from build123d import *

# Parameters (mm, degrees)
SKETCH_1_R               = 70
EXTRUDE_1_DEPTH          = 10
SKETCH_3_R               = 105
SKETCH_3_R_2             = 70
EXTRUDE_3_DEPTH          = 30
SKETCH_6_R               = 34
EXTRUDE_4_DEPTH          = 10
SKETCH_7_R               = 22
CUT_EXTRUDE_1_DEPTH      = 30
CUT_EXTRUDE_2_DEPTH      = 20
PATTERN_CIRCULAR_1_COUNT = 6
SKETCH_10_R              = 3
CUT_EXTRUDE_4_DEPTH      = 30
PATTERN_CIRCULAR_2_COUNT = 4
SKETCH_15_R              = 34
CUT_EXTRUDE_6_DEPTH      = 5


with BuildPart() as part:
    # 草图1 → 凸台-拉伸1 (new, symmetric)
    with BuildSketch(Plane(origin=(0, 0, 0), x_dir=(1, 0, 0), z_dir=(0, 1, 0))):
        with Locations(Location((0, 0, 0), (0, 0, 270))):
            Circle(SKETCH_1_R)
    extrude(amount=EXTRUDE_1_DEPTH, both=True)

    # 草图3 → 凸台-拉伸3 (add, symmetric)
    with BuildSketch(Plane(origin=(0, 0, 0), x_dir=(1, 0, 0), z_dir=(0, 1, 0))):
        with Locations(Location((0, 0, 0), (0, 0, 270))):
            Circle(SKETCH_3_R)
        with Locations(Location((0, 0, 0), (0, 0, 270))):
            Circle(SKETCH_3_R_2, mode=Mode.SUBTRACT)
    extrude(amount=EXTRUDE_3_DEPTH, both=True)

    # 草图6 → 凸台-拉伸4 (add)
    with BuildSketch(Plane.XZ.offset(10)):
        with Locations(Location((0, 0, 0), (0, 0, 90))):
            Circle(SKETCH_6_R)
    extrude(amount=EXTRUDE_4_DEPTH)

    # 草图7 → 切除-拉伸1 (cut)
    with BuildSketch(Plane.XZ.offset(20)):
        with Locations(Location((0, 0, 0), (0, 0, 270))):
            Circle(SKETCH_7_R)
    extrude(amount=-CUT_EXTRUDE_1_DEPTH, mode=Mode.SUBTRACT)

    # 草图8 → 切除-拉伸2 (cut)
    with BuildSketch(Plane.XZ.offset(10)):
        with BuildLine():
            Line((-6.945927107, 39.39231012), (-11.287131548, 64.012503946))
            ThreePointArc((-11.287131548, 64.012503946), (0, 65), (11.287131548, 64.012503946))
            Line((11.287131548, 64.012503946), (6.945927107, 39.39231012))
            ThreePointArc((6.945927107, 39.39231012), (0, 40), (-6.945927107, 39.39231012))
        make_face()
    cut_extrude_2 = extrude(amount=-CUT_EXTRUDE_2_DEPTH, mode=Mode.SUBTRACT)

    # 阵列(圆周)1: 切除-拉伸2 ×6 about axis
    pattern_circular_1_axis = Axis((0, 0, 0), (0, 1, 0))
    for i in range(1, PATTERN_CIRCULAR_1_COUNT):
        add(cut_extrude_2.rotate(pattern_circular_1_axis, i * 360 / PATTERN_CIRCULAR_1_COUNT), mode=Mode.SUBTRACT)

    # 草图10 → 切除-拉伸4 (cut)
    with BuildSketch(Plane(origin=(0, 10, 0), x_dir=(1, 0, 0), z_dir=(0, 1, 0))):
        with Locations(Location((0, 28, 0), (0, 0, 270))):
            Circle(SKETCH_10_R)
    cut_extrude_4 = extrude(amount=-CUT_EXTRUDE_4_DEPTH, mode=Mode.SUBTRACT)

    # 阵列(圆周)2: 切除-拉伸4 ×4 about axis
    pattern_circular_2_axis = Axis((0, 0, 0), (0, 1, 0))
    for i in range(1, PATTERN_CIRCULAR_2_COUNT):
        add(cut_extrude_4.rotate(pattern_circular_2_axis, i * 360 / PATTERN_CIRCULAR_2_COUNT), mode=Mode.SUBTRACT)

    # 草图15 → 切除-拉伸6 (cut)
    with BuildSketch(Plane(origin=(0, 10, 0), x_dir=(1, 0, 0), z_dir=(0, 1, 0))):
        with Locations(Location((0, 0, 0), (0, 0, 270))):
            Circle(SKETCH_15_R)
    extrude(amount=-CUT_EXTRUDE_6_DEPTH, mode=Mode.SUBTRACT)


solid = part.part
Part model, mm, in its own coordinate system. A direction names the side the tool comes from. Give positions to 0.01 mm unless a question says otherwise; leave off trailing zeros. Order: outer loops, then holes, each group sorted by start corner. A loop starts at its lowest first (then second) coordinate and runs counter-clockwise, first axis right, second up. Notation, with made-up numbers: (12.5, 13) - (29.5, 13) arc R22 cw to (29.5, 42) - close; hole circle Ø4 at (74.5, 61.5). An arc over 180 degrees is marked (long way). Use a Markdown table: item, result.
1) 3-axis set-ups, long thin cutter, end or side, ignore diameter. For faces 3 (the cylindrical face through (-42.594, 19.86, -55.55)), 4 (the cylindrical face through (56, 0, 33)), 5 (the cylindrical face through (-33.71, -14.93, -4.43)): which of +Z, -Z, +X, -X, +Y, -Y reach the whole face in a straight line?
Checked values:
| item | result |
|---|---|
| face 3 | +Y |
| face 4 | +Y, -Y |
| face 5 | -Y |
2) Flat gauge pins, fed straight in: P1, Ø6, axis at y = -6.5, z = -74.5, coming from the -X side; P2, Ø1.5, axis at x = 13.5, z = -34.5, coming from the +Y side; P3, Ø8, axis at x = 0, z = -28, coming from the +Y side; P4, Ø5, axis at x = 6.5, z = 53, coming from the +Y side. Where does each tip first touch, or does it go through?
Checked values:
| item | result |
|---|---|
| P1 | x = -76.89 |
| P2 | y = 10 |
| P3 | y = 5 |
| P4 | through |
3) Probe L1, parallel to X at y = 21.5, z = 0; L2, parallel to X at y = 7, z = 27; L3, parallel to X at y = 24.5, z = -2.5. List the from-to ranges inside material, lowest first. Write a range as from..to.
Checked values:
| item | result |
|---|---|
| L1 | -105..-70, 70..105 |
| L2 | -101.47..-59.13, -32.18..-20.66, 20.66..32.18, 59.13..101.47 |
| L3 | -104.97..-69.96, 69.96..104.97 |
4) Saw through at A-A on y = -3. Count the separate pieces of the cut face and the enclosed holes in it, plus the area to 3 significant figures.
Checked values:
| item | result |
|---|---|
| separate pieces | 1 |
| enclosed holes | 11 |
| area | 30,300 mm² |
5) Two-plate mould, pull along X, no slides. Class faces 1 (the cylindrical face through (33.71, 7.54, -4.43)), 2 (the cylindrical face through (31.54, 0.42, 100.15)): +X half, -X half, draft (parallel to the pull), parting line (faces both ways), or undercut.
Checked values:
| item | result |
|---|---|
| face 1 | undercut |
| face 2 | parting line |
6) Saw through at C-C on x = -28. List the corners of the cut face in (y, z), plus the area to 3 significant figures.
Checked values:
| item | result |
|---|---|
| outline | (-30, -101.2) - (30, -101.2) - (30, -64.16) - (10, -64.16) - (10, -19.29) - (5, -19.29) - (5, -3) - (-20, -3) - (-20, -19.29) - (-10, -19.29) - (-10, -64.16) - (-30, -64.16) - close; (-30, 64.16) - (-10, 64.16) - (-10, 19.29) - (-20, 19.29) - (-20, 3) - (5, 3) - (5, 19.29) - (10, 19.29) - (10, 64.16) - (30, 64.16) - (30, 101.2) - (-30, 101.2) - close |
| area | 7,050 mm² |
